Here's how the part is built. I have some questions about the finished solid (model axes, mm). Face numbers are marked on the shaded views. A direction names the side the tool comes from. Round coordinates to 2 decimals unless told otherwise and drop trailing zeros. Order: outer loops, then holes, each group sorted by start corner. A loop starts at its lowest first (then second) coordinate and runs counter-clockwise, first axis right, second up. Notation, with made-up numbers: M -6,16.25 L 42,16.25 A17 cw 42,37.25 Z; hole C 86,87 d3. An arc over 180 degrees is marked long. Write item = value, one per line. Start each with the question number.
Item 1: I want a section at B-B, the plane x = 0. List the corners of the cut face in (y, z) for me, plus the area to 3 significant figures.
Item 2: Please list where these lines run through material, in increasing order: L1, parallel to Z at x = 0.4, y = 0; L2, parallel to Y at x = -0.5, z = 26; L3, parallel to Z at x = 1.25, y = -2.5.
Item 3: I want a section at C-C, the plane z = 11.25. List the corners of the cut face in (x, y) for me, plus the area to 3 significant figures.
Item 4: I want a section at A-A, the plane y = 0. List the corners of the cut face in (x, z) for me.
Item 5: I'm going to push flat-ended pins straight in: P1, Ø1, axis at y = -3.5, z = 18, coming from the -X side; P2, Ø4, axis at x = 1.5, z = 14.5, coming from the -Y side; P3, Ø2, axis at x = 1.5, y = 1.5, coming from the +Z side; P4, Ø1.5, axis at y = -2.5, z = 8, coming from the +X side. Where does each tip first touch, or does it pass through?
Item 6: I want a section at D-D, the plane z = 26. List the corners of the cut face in (x, y) for me, plus the area to 3 significant figures.
Item 7: For the marked faces 1 and 2, which set-ups out of +Z, -Z, +X, -X, +Y, -Y let a thin tool reach every point of the face, with its end or its side?
```python
from build123d import *

# Parameters (mm, degrees)
F0_R        = 5
F1_DEPTH    = 10
F2_R        = 1.5
F3_DEPTH    = 16
F7_SIZE     = 1
F8_DEPTH    = 12.5
F9_T2_ANGLE = 245.2760469103
F9_T4_ANGLE = 245.2760469103


# Not quite as in the source:
# - a fillet or chamfer that OpenCascade refuses, or shapes differently, is made with other operations: its cross-section is extruded or revolved along the edge and cut away or added


with BuildPart() as f1:
    # F0 (on Top) → F1 (new body)
    with BuildSketch(Plane.XY):
        Circle(F0_R)
    extrude(amount=F1_DEPTH)

    # F2 (on face) → F3 (join)
    with BuildSketch(Plane.XY.offset(10)):
        Circle(F2_R)
    extrude(amount=F3_DEPTH)

    # F4 (on Right) → F5 (revolve)
    with BuildSketch(Plane.YZ):
        with BuildLine():
            ThreePointArc((1.5, 26), (0, 27.5), (-1.5, 26))
            Line((-1.5, 26), (1.5, 26))
        make_face()
    revolve(axis=Axis((0, 0, 26), (0, 1, 0)))

    # F7
    f7_edges = [f1.edges().sort_by_distance(p)[0] for p in [
        (-5, 0, 10),
        (-1.5, 0, 10),
    ]]
    chamfer(f7_edges, length=F7_SIZE)

    # F6 (on Right) → F8 (cut, symmetric)
    with BuildSketch(Plane.YZ):
        with BuildLine():
            Line((-1.4142135624, 26.5), (-0.9797958971, 26.5))
            ThreePointArc((-0.9797958971, 26.5), (0, 24.9), (0.9797958971, 26.5))
            Line((0.9797958971, 26.5), (1.4142135624, 26.5))
            ThreePointArc((1.4142135624, 26.5), (0, 27.5), (-1.4142135624, 26.5))
        make_face()
    extrude(amount=F8_DEPTH, both=True, mode=Mode.SUBTRACT)

    # F9: fillet of radius 0.75 on 2 edges, made by hand

    # F9_s1 → F9_t2 (revolve, cut)
    with BuildSketch(Plane(origin=(0, 0, 0), x_dir=(0, 0, 1), z_dir=(0.5393297468, -0.8420946646, 0))):
        with BuildLine():
            ThreePointArc((25.75, 1.5), (26.2803300859, 1.2803300859), (26.5, 0.75))
            Line((26.5, 0.75), (26.575, 0.75))
            Line((26.575, 0.75), (26.575, 1.4142135624))
            Line((26.575, 1.4142135624), (26.525, 1.4849242405))
            ThreePointArc((26.525, 1.4849242405), (26, 1.575), (25.75, 1.575))
            Line((25.75, 1.575), (25.75, 1.5))
        make_face()
    revolve(axis=Axis((0, 0, 26.5), (0, 0, -1)), revolution_arc=F9_T2_ANGLE, mode=Mode.SUBTRACT)

    # F9_s3 → F9_t4 (revolve, cut)
    with BuildSketch(Plane(origin=(0, 0, 0), x_dir=(0, 0, 1), z_dir=(-0.5393297468, 0.8420946646, 0))):
        with BuildLine():
            ThreePointArc((25.75, 1.5), (26.2803300859, 1.2803300859), (26.5, 0.75))
            Line((26.5, 0.75), (26.575, 0.75))
            Line((26.575, 0.75), (26.575, 1.4142135624))
            Line((26.575, 1.4142135624), (26.525, 1.4849242405))
            ThreePointArc((26.525, 1.4849242405), (26, 1.575), (25.75, 1.575))
            Line((25.75, 1.575), (25.75, 1.5))
        make_face()
    revolve(axis=Axis((0, 0, 26.5), (0, 0, -1)), revolution_arc=F9_T4_ANGLE, mode=Mode.SUBTRACT)


solid = f1.part
```
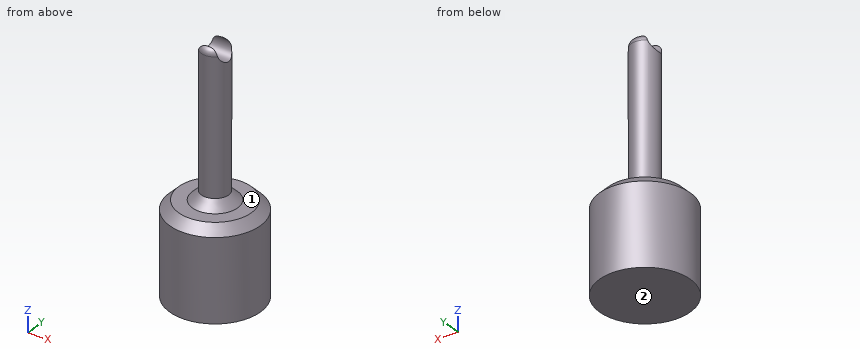
Filled in:
q1.outline = M -5,0 L 5,0 L 5,9 L 4,10 L 2.5,10 L 1.5,11 L 1.5,25.75 A0.75 ccw 1,26.46 A1.1 cw long -1,26.46 A0.75 ccw -1.5,25.75 L -1.5,11 L -2.5,10 L -4,10 L -5,9 Z
q1.area = 146 mm^2
q2.L1 = 0 to 24.9
q2.L2 = -1.37 to -1.1, 1.1 to 1.37
q2.L3 = 0 to 10
q3.outline = C 0,0 d3
q3.area = 7.07 mm^2
q4.outline = M -5,0 L 5,0 L 5,9 L 4,10 L 2.5,10 L 1.5,11 L 1.5,24.9 L -1.5,24.9 L -1.5,11 L -2.5,10 L -4,10 L -5,9 Z
q5.P1 = through
q5.P2 = -1.5
q5.P3 = 26.34
q5.P4 = 4.68
q6.outline = M -0.96,-1.1 A1.46 ccw 0.96,-1.1 Z; M -0.96,1.1 L 0.96,1.1 A1.46 ccw Z
q6.area = 0.935 mm^2
q7.face_1 = +Z
q7.face_2 = -Z, +X, -X, +Y, -Y
